```python
from build123d import *

# Parameters (mm, degrees)
SKETCH3_R            = 27.94
BOSS_EXTRUDE2_DEPTH  = 122.46
SKETCH5_R            = 3.175
CUT_EXTRUDE1_DEPTH   = 129.676877488
SKETCH4_W            = 14
SKETCH4_H            = 6
SHELL1_START         = 3
SHELL1_OUTLINE_R     = 10.94
SHELL1_OUTLINE_R_2   = 6.175
SHELL1_DEPTH         = 116.46
SHELL1_2_OUTLINE_R   = 24.94
SHELL1_2_OUTLINE_R_2 = 10.94
SHELL1_2_DEPTH       = 10.72
SHELL1_START_2       = 109.72
SHELL1_3_OUTLINE_R   = 24.94
SHELL1_3_OUTLINE_R_2 = 10.94
SHELL1_3_DEPTH       = 9.74
SHELL1_START_3       = 25.72
SHELL1_4_OUTLINE_R   = 24.94
SHELL1_4_OUTLINE_R_2 = 10.94
SHELL1_4_DEPTH       = 9
SHELL1_START_4       = 46.72
SHELL1_5_OUTLINE_R   = 24.94
SHELL1_5_OUTLINE_R_2 = 10.94
SHELL1_5_DEPTH       = 9
SHELL1_START_5       = 67.72
SHELL1_6_OUTLINE_R   = 24.94
SHELL1_6_OUTLINE_R_2 = 10.94
SHELL1_6_DEPTH       = 9
SHELL1_START_6       = 88.72
SHELL1_7_OUTLINE_R   = 24.94
SHELL1_7_OUTLINE_R_2 = 10.94
SHELL1_7_DEPTH       = 9
BOSS_EXTRUDE3_REACH  = 130.677
SKETCH13_W           = 16.483162312
SKETCH13_H           = 6
CUT_EXTRUDE3_DEPTH   = 123
BOSS_EXTRUDE5_START  = -122.46
BOSS_EXTRUDE5_DEPTH  = 122.46


# Read off the part's stored shape, not the designer's step: Shell1
with BuildPart() as part:
    # Sketch3 → Boss-Extrude2 (new body)
    with BuildSketch(Plane.XY):
        Circle(SKETCH3_R)
    extrude(amount=BOSS_EXTRUDE2_DEPTH)

    # Sketch5 → Cut-Extrude1 (cut, through all)
    with BuildSketch(Plane.XY.offset(122.46)):
        Circle(SKETCH5_R)
    extrude(amount=-CUT_EXTRUDE1_DEPTH, mode=Mode.SUBTRACT)

    # Sketch4 → Cut-Revolve1 (revolve, cut)
    with BuildSketch(Plane(origin=(0, 0, 0), x_dir=(1, 0, 0), z_dir=(0, 1, 0)), mode=Mode.PRIVATE) as cut_revolve1_sk:
        with Locations((-20.94, -103.72)):
            Rectangle(SKETCH4_W, SKETCH4_H)
        with Locations((-20.94, -82.72)):
            Rectangle(SKETCH4_W, SKETCH4_H)
        with Locations((-20.94, -61.72)):
            Rectangle(SKETCH4_W, SKETCH4_H)
        with Locations((-20.94, -40.72)):
            Rectangle(SKETCH4_W, SKETCH4_H)
        with Locations((-20.94, -19.72)):
            Rectangle(SKETCH4_W, SKETCH4_H)
    revolve(cut_revolve1_sk.sketch.rotate(Axis((0, 0, 122.46), (0, 0, -1)), 180), axis=Axis((0, 0, 122.46), (0, 0, -1)), mode=Mode.SUBTRACT)

    # Shell1 outline → Shell1 (cut)
    with BuildSketch(Plane.XY.offset(SHELL1_START)):
        Circle(SHELL1_OUTLINE_R)
        Circle(SHELL1_OUTLINE_R_2, mode=Mode.SUBTRACT)
    extrude(amount=SHELL1_DEPTH, mode=Mode.SUBTRACT)

    # Shell1 2 outline → Shell1 2 (cut)
    with BuildSketch(Plane.XY.offset(SHELL1_START)):
        Circle(SHELL1_2_OUTLINE_R)
        Circle(SHELL1_2_OUTLINE_R_2, mode=Mode.SUBTRACT)
    extrude(amount=SHELL1_2_DEPTH, mode=Mode.SUBTRACT)

    # Shell1 3 outline → Shell1 3 (cut)
    with BuildSketch(Plane.XY.offset(SHELL1_START_2)):
        Circle(SHELL1_3_OUTLINE_R)
        Circle(SHELL1_3_OUTLINE_R_2, mode=Mode.SUBTRACT)
    extrude(amount=SHELL1_3_DEPTH, mode=Mode.SUBTRACT)

    # Shell1 4 outline → Shell1 4 (cut)
    with BuildSketch(Plane.XY.offset(SHELL1_START_3)):
        Circle(SHELL1_4_OUTLINE_R)
        Circle(SHELL1_4_OUTLINE_R_2, mode=Mode.SUBTRACT)
    extrude(amount=SHELL1_4_DEPTH, mode=Mode.SUBTRACT)

    # Shell1 5 outline → Shell1 5 (cut)
    with BuildSketch(Plane.XY.offset(SHELL1_START_4)):
        Circle(SHELL1_5_OUTLINE_R)
        Circle(SHELL1_5_OUTLINE_R_2, mode=Mode.SUBTRACT)
    extrude(amount=SHELL1_5_DEPTH, mode=Mode.SUBTRACT)

    # Shell1 6 outline → Shell1 6 (cut)
    with BuildSketch(Plane.XY.offset(SHELL1_START_5)):
        Circle(SHELL1_6_OUTLINE_R)
        Circle(SHELL1_6_OUTLINE_R_2, mode=Mode.SUBTRACT)
    extrude(amount=SHELL1_6_DEPTH, mode=Mode.SUBTRACT)

    # Shell1 7 outline → Shell1 7 (cut)
    with BuildSketch(Plane.XY.offset(SHELL1_START_6)):
        Circle(SHELL1_7_OUTLINE_R)
        Circle(SHELL1_7_OUTLINE_R_2, mode=Mode.SUBTRACT)
    extrude(amount=SHELL1_7_DEPTH, mode=Mode.SUBTRACT)

    # Boss-Extrude3: up to this face of the body (flat: up to its plane)
    boss_extrude3_end = Plane(part.part.faces().sort_by_distance((-27.149737461, 0, 122.46))[0])
    # Sketch10 → Boss-Extrude3 (add, up to the picked face)
    with BuildSketch(Plane(origin=(0, 0, 0), x_dir=(-1, 0, 0), z_dir=(0, 0, -1)), mode=Mode.PRIVATE) as boss_extrude3_sk1:
        with BuildLine():
            Line((-1, 27.922098775), (-1, 3.01340754))
            ThreePointArc((-1, 3.01340754), (0, 3.175), (1, 3.01340754))
            Line((1, 3.01340754), (1, 27.922098775))
            ThreePointArc((1, 27.922098775), (0, 27.94), (-1, 27.922098775))
        make_face()
    boss_extrude3_tool1 = split(extrude(boss_extrude3_sk1.sketch, amount=-BOSS_EXTRUDE3_REACH, mode=Mode.PRIVATE), bisect_by=boss_extrude3_end, keep=Keep.BOTH, mode=Mode.PRIVATE)
    # Sketch10 → Boss-Extrude3 (add, up to the picked face)
    with BuildSketch(Plane(origin=(0, 0, 0), x_dir=(-1, 0, 0), z_dir=(0, 0, -1)), mode=Mode.PRIVATE) as boss_extrude3_sk2:
        with BuildLine():
            Line((3.01340754, 1), (27.922098775, 1))
            ThreePointArc((27.922098775, 1), (27.94, 0), (27.922098775, -1))
            Line((27.922098775, -1), (3.01340754, -1))
            ThreePointArc((3.01340754, -1), (3.175, 0), (3.01340754, 1))
        make_face()
    boss_extrude3_tool2 = split(extrude(boss_extrude3_sk2.sketch, amount=-BOSS_EXTRUDE3_REACH, mode=Mode.PRIVATE), bisect_by=boss_extrude3_end, keep=Keep.BOTH, mode=Mode.PRIVATE)
    # Sketch10 → Boss-Extrude3 (add, up to the picked face)
    with BuildSketch(Plane(origin=(0, 0, 0), x_dir=(-1, 0, 0), z_dir=(0, 0, -1)), mode=Mode.PRIVATE) as boss_extrude3_sk3:
        with BuildLine():
            Line((-1, -3.01340754), (-1, -27.922098775))
            ThreePointArc((-1, -27.922098775), (0, -27.94), (1, -27.922098775))
            Line((1, -27.922098775), (1, -3.01340754))
            ThreePointArc((1, -3.01340754), (0, -3.175), (-1, -3.01340754))
        make_face()
    boss_extrude3_tool3 = split(extrude(boss_extrude3_sk3.sketch, amount=-BOSS_EXTRUDE3_REACH, mode=Mode.PRIVATE), bisect_by=boss_extrude3_end, keep=Keep.BOTH, mode=Mode.PRIVATE)
    # Sketch10 → Boss-Extrude3 (add, up to the picked face)
    with BuildSketch(Plane(origin=(0, 0, 0), x_dir=(-1, 0, 0), z_dir=(0, 0, -1)), mode=Mode.PRIVATE) as boss_extrude3_sk4:
        with BuildLine():
            Line((-27.922098775, -1), (-3.01340754, -1))
            ThreePointArc((-3.01340754, -1), (-3.175, 0), (-3.01340754, 1))
            Line((-3.01340754, 1), (-27.922098775, 1))
            ThreePointArc((-27.922098775, 1), (-27.94, 0), (-27.922098775, -1))
        make_face()
    boss_extrude3_tool4 = split(extrude(boss_extrude3_sk4.sketch, amount=-BOSS_EXTRUDE3_REACH, mode=Mode.PRIVATE), bisect_by=boss_extrude3_end, keep=Keep.BOTH, mode=Mode.PRIVATE)
    add(boss_extrude3_tool1.solids().sort_by(Axis((0, 15.527819, 0), (0, 0, 1)))[0])
    add(boss_extrude3_tool2.solids().sort_by(Axis((-15.527819, 0, 0), (0, 0, 1)))[0])
    add(boss_extrude3_tool3.solids().sort_by(Axis((0, -15.527819, 0), (0, 0, 1)))[0])
    add(boss_extrude3_tool4.solids().sort_by(Axis((15.527819, 0, 0), (0, 0, 1)))[0])

    # Sketch13 → Cut-Revolve2 (revolve, cut)
    with BuildSketch(Plane(origin=(0, 0, 0), x_dir=(1, 0, 0), z_dir=(0, 1, 0)), mode=Mode.PRIVATE) as cut_revolve2_sk:
        with Locations((-22.145666886, -40.72)):
            Rectangle(SKETCH13_W, SKETCH13_H)
        with Locations((-22.145666886, -19.72)):
            Rectangle(SKETCH13_W, SKETCH13_H)
        with Locations((-22.145666886, -61.72)):
            Rectangle(SKETCH13_W, SKETCH13_H)
        with Locations((-22.145666886, -82.72)):
            Rectangle(SKETCH13_W, SKETCH13_H)
        with Locations((-22.145666886, -103.72)):
            Rectangle(SKETCH13_W, SKETCH13_H)
    revolve(cut_revolve2_sk.sketch.rotate(Axis((0, 0, 121.588746248), (0, 0, -1)), 180), axis=Axis((0, 0, 121.588746248), (0, 0, -1)), mode=Mode.SUBTRACT)

    # Sketch16 → Cut-Extrude3 (cut)
    with BuildSketch(Plane(origin=(0, 0, 0), x_dir=(-1, 0, 0), z_dir=(0, 0, -1))):
        with BuildLine():
            Line((-27.923120749, -0.971044624), (-6.098171639, -0.971044624))
            ThreePointArc((-6.098171639, -0.971044624), (-0.014665674, -6.174982584), (6.093490379, -1))
            Line((6.093490379, -1), (27.922098775, -1))
            ThreePointArc((27.922098775, -1), (-0.014486703, -27.939996244), (-27.923120749, -0.971044624))
        make_face()
    extrude(amount=-CUT_EXTRUDE3_DEPTH, mode=Mode.SUBTRACT)

    # Sketch18 → Boss-Extrude5 (add)
    with BuildSketch(Plane(origin=(0, 0, 0), x_dir=(-1, 0, 0), z_dir=(0, 0, -1)).offset(BOSS_EXTRUDE5_START)):
        with BuildLine():
            Line((-3.175, 0), (-9.175, 0))
            ThreePointArc((-9.175, 0), (0, -9.175), (9.175, 0))
            Line((9.175, 0), (3.175, 0))
            ThreePointArc((3.175, 0), (0, -3.175), (-3.175, 0))
        make_face()
    extrude(amount=BOSS_EXTRUDE5_DEPTH)


solid = part.part
```
Geometry check sheet. Reference: the model listing, model coordinates, mm. A direction names the side the tool comes from. Coordinates: 2 decimals unless noted, no trailing zeros. Answer as a JSON object with one key per item and string values.
Q1. Release check for a two-part mould opening along X. For faces 3 (the flat face through (-13, 13, 13.72)), 4 (the flat face through (0, 16, 43.72)), 5 (the cylindrical face through (-0.3, 13.9, 19.7)) record: released by +X, released by -X, zero draft, split by the parting line, or undercut.
Results are:
{"face 3": "undercut", "face 4": "zero draft", "face 5": "split by the parting line"}
Q2. Depth check by flat-ended pin: pin 1 Ø6 at (x, z) = (12, 93) entering from +Y; pin 2 Ø12 at (x, z) = (-6.5, 66.5) entering from -Y; pin 3 Ø5.5 at (x, z) = (-18.5, 91.5) entering from -Y. Enter the tip coordinate at first touch or a pass-through.
Results are:
{"pin 1": "stops at y = 26.45", "pin 2": "stops at y = -9.16", "pin 3": "stops at y = -1"}
Q3. Scan lines: line 1 (Z direction, x = -6, y = 26.5); line 2 (X direction, y = 0, z = 92) (3 decimals); line 3 (Z direction, x = 6, y = 8). Record each from-to range of solid material in increasing order.
Results are:
{"line 1": "z = 0 to 16.72, 22.72 to 37.72, 43.72 to 58.72, 64.72 to 79.72, 85.72 to 100.72, 106.72 to 122.46", "line 2": "x = -27.94 to -3.175, 3.175 to 27.94", "line 3": "z = 0 to 3, 119.46 to 122.46"}
Q4. Cross-section at A-A on z = 91.5. Give the number of separate pieces and of enclosed holes in the cut face, and give its area (3 significant figures).
Results are:
{"separate pieces": "1", "enclosed holes": "3", "area": "522 mm²"}
Q5. Tool access check on faces 1 (the flat face through (13, 13, 46.72)), 2 (the flat face through (-12, -1, 60)). Record the directions out of +Z, -Z, +X, -X, +Y, -Y that give a thin tool (end or side, any length) a straight path to the whole face; none if there is none.
Results are:
{"face 1": "none", "face 2": "+Z, -Z, -X, -Y"}
